Build history of the part. All positions in model axes, mm. A direction names the side the tool comes from. Round coordinates to 2 decimals unless told otherwise and drop trailing zeros. Order: outer loops, then holes, each group sorted by start corner. A loop starts at its lowest first (then second) coordinate and runs counter-clockwise, first axis right, second up. Notation, with made-up numbers: (-30.5, 9) -> (-8.5, 9) arc R37 ccw to (-8.5, 48) -> close; hole circle Ø6 at (77.5, -1.75). An arc over 180 degrees is marked (long way). Answer as a JSON object with one key per item and string values.
from build123d import *

# Parameters (mm, degrees)
F1_DEPTH = 25


with BuildPart() as f1:
    # F0 (on Front) → F1 (new body)
    with BuildSketch(Plane.XZ):
        Polygon((-89.9047479033, 42.2662571073), (-35.2840051055, 32.0440493524), (56.9544807076, 32.0440493524), (70.2112689614, 44.4089584053), (42.0486187137, 44.4089584053), (-89.9047479033, 44.4089584053), align=None)
        Polygon((70.2112689614, 44.4089584053), (56.9544807076, 32.0440493524), (40.7549355767, 10.6797787951), (70.2112689614, -24.8387977481), align=None)
        Polygon((-65.2892962098, -18.5195934027), (-39.2996874644, 25.2769919188), (-89.9047479033, 26.4464366573), (-89.9047479033, -24.8387977481), align=None)
        Polygon((-181.8143725395, 28.5703986883), (-89.9047479033, 42.2662571073), (-89.9047479033, 44.4089584053), (-181.0087710619, 127.9826015234), align=None)
        Polygon((-89.9047479033, 26.4464366573), (-89.9047479033, 42.2662571073), (-181.8143725395, 28.5703986883), align=None)
        Polygon((70.2112689614, -24.8387977481), (40.7549355767, 10.6797787951), (18.6143927276, -18.5195934027), align=None)
        Polygon((42.0486187137, 44.4089584053), (70.2112689614, 44.4089584053), (24.6596280485, 93.4770107269), (-122.2022771835, 93.4770107269), (-89.9047479033, 69.2056491971), (12.4589074403, 69.2056491971), align=None)
        Polygon((24.6596280485, 93.4770107269), (70.2112689614, 44.4089584053), (39.0130095184, 127.9826015234), (-181.0087710619, 127.9826015234), (-89.9047479033, 44.4089584053), (-122.2022771835, 93.4770107269), align=None)
        Polygon((18.6143927276, -18.5195934027), (-65.2892962098, -18.5195934027), (-89.9047479033, -24.8387977481), (70.2112689614, -24.8387977481), align=None)
        Polygon((-89.9047479033, -24.8387977481), (-89.9047479033, 26.4464366573), (-181.8143725395, 28.5703986883), align=None)
    extrude(amount=F1_DEPTH)


solid = f1.part
1) Cut at D-D, the plane x = 50. Give the cut face in (y, z).
Checked values:
{"outline": "(-25, -24.84) -> (0, -24.84) -> (0, 22.87) -> (-25, 22.87) -> close; (-25, 32.04) -> (0, 32.04) -> (0, 98.55) -> (-25, 98.55) -> close"}
2) Cut at A-A, the plane x = -22. Give the cut face in (y, z).
Checked values:
{"outline": "(-25, -24.84) -> (0, -24.84) -> (0, -18.52) -> (-25, -18.52) -> close; (-25, 32.04) -> (0, 32.04) -> (0, 44.41) -> (-25, 44.41) -> close; (-25, 69.21) -> (0, 69.21) -> (0, 127.98) -> (-25, 127.98) -> close"}
3) Pull direction Z, two halves, no side cores. Call faces 3 (the face through (-58, -25, 70)), 4 (the face through (-62.977, -12.325, 37.227)), 5 (the face through (54.83, -12.32, 85.61)): pulls with the +Z half, pulls with the -Z half, needs draft (parallel to the pull), parting line crosses it, or undercut.
Checked values:
{"face 3": "needs draft", "face 4": "undercut", "face 5": "pulls with the +Z half"}
4) Cut at C-C, the plane z = 4. Give the cut face in (x, y), plus the area to 3 significant figures.
Checked values:
{"outline": "(-139.53, -25) -> (-51.93, -25) -> (-51.93, 0) -> (-139.53, 0) -> close; (35.69, -25) -> (70.21, -25) -> (70.21, 0) -> (35.69, 0) -> close", "area": "3,050 mm²"}
5) Flat gauge pins, fed straight in: pin 1 Ø1 at (y, z) = (-16, 49.5) entering from +X; pin 2 Ø1 at (x, y) = (-119.5, -8) entering from -Z; pin 3 Ø12 at (x, y) = (-106, -5.5) entering from -Z. Where does each tip first touch, or does it go through?
Checked values:
{"pin 1": "stops at x = 68.5", "pin 2": "stops at z = -7.93", "pin 3": "stops at z = -18.97"}
6) Which spindle directions (+Z, -Z, +X, -X, +Y, -Y) get a long thin tool onto all of the face, cutting with end or side? Do faces 1 (the face through (-69, -12, 127.983)), 2 (the face through (10, -12, 32.044)). Say none if no direction does.
Checked values:
{"face 1": "+Z, +X, -X, +Y, -Y", "face 2": "+Y, -Y"}
7) Probe L1, parallel to Z at x = 6, y = -10.25; L2, parallel to Z at x = 23, y = -19.5; L3, parallel to Z at x = -47, y = -2. List the from-to ranges inside material, lowest first. Write a range as from..to.
Checked values:
{"L1": "z = -24.84..-18.52, 32.04..44.41, 69.21..127.98", "L2": "z = -24.84..-12.74, 32.04..44.41, 60.37..127.98", "L3": "z = -24.84..-18.52, 12.3..25.45, 34.24..44.41, 69.21..127.98"}
8) Cut at B-B, the plane y = -18.5. Give the cut face in (x, z).
Checked values:
{"outline": "(-181.81, 28.57) -> (-89.9, -24.84) -> (70.21, -24.84) -> (70.21, 44.41) -> (39.01, 127.98) -> (-181.01, 127.98) -> close; hole (-122.2, 93.48) -> (-89.9, 44.41) -> (42.05, 44.41) -> (12.46, 69.21) -> (-89.9, 69.21) -> close; hole (-89.9, 26.45) -> (-39.3, 25.28) -> (-65.29, -18.52) -> (18.61, -18.52) -> (56.95, 32.04) -> (-35.28, 32.04) -> (-89.9, 42.27) -> close"}
